```python
from build123d import *

# Parameters (mm, degrees)
F1_DEPTH       = 32
F3_D           = 3
F3_DEPTH       = 40
F3_CBORE_D     = 3
F3_CBORE_DEPTH = 40
F3_TIP         = 0.9012909285
F4_DEPTH       = 10
F6_DEPTH       = 2.6


with BuildPart() as f1:
    # F0 (on Top) → F1 (new body)
    with BuildSketch(Plane.XY):
        Polygon((-5.9322740159, -3.425), (0, -6.85), (5.9322740159, -3.425), (5.9322740159, 3.425), (0, 6.85), (-5.9322740159, 3.425), align=None)
    extrude(amount=F1_DEPTH)

    # F3
    with Locations(Plane.XY.offset(32)):
        with Locations((0, 0)):
            CounterBoreHole(F3_D / 2, F3_CBORE_D / 2, F3_CBORE_DEPTH, depth=F3_DEPTH)
            with Locations((0, 0, -(F3_DEPTH + F3_TIP / 2))):  # 118° drill point
                Cone(0, F3_D / 2, F3_TIP, mode=Mode.SUBTRACT)

    # F4 (add): a face of the model
    f4_faces = [f1.faces().sort_by_distance(p)[0] for p in [
        (-5.7510400511, 0, 32),
    ]]
    extrude(f4_faces, amount=F4_DEPTH)

    # F5 (on face) → F6 (cut)
    with BuildSketch(Plane.XY.offset(42)):
        Polygon((1.6454482672, 2.85), (-1.6454482672, 2.85), (-3.2908965344, 0), (-1.6454482672, -2.85), (1.6454482672, -2.85), (3.2908965344, 0), align=None)
    extrude(amount=-F6_DEPTH, mode=Mode.SUBTRACT)


solid = f1.part
```
Work out the finished part from the listing and answer in its coordinate system (mm). A direction names the side the tool comes from. Give positions to 0.01 mm unless a question says otherwise; leave off trailing zeros. Write each loop counter-clockwise with the first axis right and the second up, starting at its lowest first coordinate (ties: lowest second). Pieces come first, ordered by that corner, then holes.
(1) Straight lines are drawn through the part: line 1 (X direction, y = 0, z = 21); line 2 (Y direction, x = 0, z = 21); line 3 (Y direction, x = -0.5, z = 37). For each, find the intervals that lie inside material, in ascending order.
Final values:
line 1: x = -5.93 to -1.5, 1.5 to 5.93
line 2: y = -6.85 to -1.5, 1.5 to 6.85
line 3: y = -6.56 to -1.41, 1.41 to 6.56
(2) The part is cut by section D-D on y = 5. Write down the section's boundary in (x, z), plus the area to 3 significant figures.
Final values:
outline: (-3.2, 0) - (3.2, 0) - (3.2, 42) - (-3.2, 42) - close
area: 269 mm2
(3) The part is cut by section B-B on z = 35. Write down the section's boundary in (x, y) (3 decimals), plus the area to 3 significant figures.
Final values:
outline: (-5.932, -3.425) - (0, -6.85) - (5.932, -3.425) - (5.932, 3.425) - (0, 6.85) - (-5.932, 3.425) - close; hole circle Ø3 at (0, 0)
area: 115 mm2
(4) Flat-ended cylindrical pins translate along their axes: pin 1 Ø4 at (x, y) = (0, 0) entering from +Z; pin 2 Ø3 at (x, z) = (0, 40) entering from +Y; pin 3 Ø1 at (x, z) = (-1.5, 8) entering from -Y. Find the tip coordinate at first contact, or state that the pin passes through.
Final values:
pin 1: stops at z = 39.4
pin 2: stops at y = 6.85
pin 3: stops at y = -6.27
(5) The part is cut by section C-C on x = 0.75. Write down the section's boundary in (y, z).
Final values:
outline: (-6.42, 0) - (-1.3, 0) - (-1.3, 39.4) - (-2.85, 39.4) - (-2.85, 42) - (-6.42, 42) - close; (1.3, 0) - (6.42, 0) - (6.42, 42) - (2.85, 42) - (2.85, 39.4) - (1.3, 39.4) - close
(6) The part is cut by section A-A on y = 0.5. Write down the section's boundary in (x, z).
Final values:
outline: (-5.93, 0) - (-1.41, 0) - (-1.41, 39.4) - (-3, 39.4) - (-3, 42) - (-5.93, 42) - close; (1.41, 0) - (5.93, 0) - (5.93, 42) - (3, 42) - (3, 39.4) - (1.41, 39.4) - close
(7) The mould has two halves that part along X. Classify faces 3 (the flat face through (-2.46, 1.44, 40.72)), 4 (the flat face through (2.925, -5.161, 20.706)), 5 (the flat face through (1.2, -1.4, 0)): pulls with the +X half, pulls with the -X half, needs draft (parallel to the pull), parting line crosses it, or undercut.
Final values:
face 3: undercut
face 4: pulls with the +X half
face 5: needs draft
(8) Which of the six approach directions +Z, -Z, +X, -X, +Y, -Y give full straight-line access (tool end or side, diameter ignored) to faces 1 (the flat face through (2.46, -1.44, 40.72)), 2 (the flat face through (-5.932, 0, 21))?
Final values:
face 1: +Z
face 2: +Z, -Z, -X, +Y, -Y
